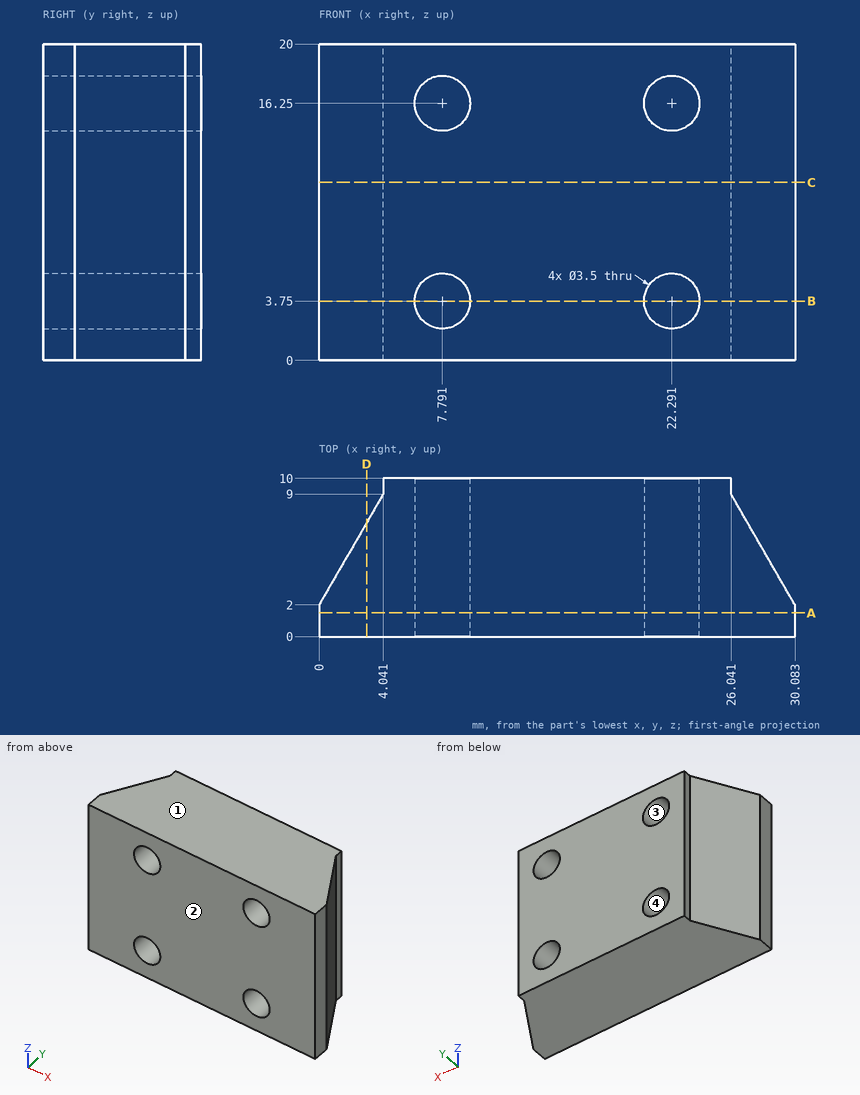
Design review of the part shown in the three views and the two pictorial views. Dimensions are in mm from the part's minimum x, y and z. Round coordinates to 2 decimals unless told otherwise and drop trailing zeros. Write each loop counter-clockwise with the first axis right and the second up, starting at its lowest first coordinate (ties: lowest second). Pieces come first, ordered by that corner, then holes.
Item 1: Consider section D-D on x = 3. Give the boundary of the cut face in (y, z), and give its area (3 significant figures).
Item 2: Consider section B-B on z = 3.75. Give the boundary of the cut face in (x, y).
Item 3: Consider section A-A on y = 1.5. Give the boundary of the cut face in (x, z).
Item 4: Consider section C-C on z = 11.25. Give the boundary of the cut face in (x, y).
Item 5: Draft analysis for pull direction Z (two halves, no side actions). For the marked faces 1, 2, 3 and 4, state which applies: released by +Z, released by -Z, zero draft, split by the parting line, or undercut.
Item 6: For pin 1 Ø3 at (x, z) = (7.79, 3.75) entering from -Y; pin 2 Ø1.1 at (y, z) = (9.5, 5.5) entering from -X; pin 3 Ø0.5 at (y, z) = (9.5, 8.5) entering from +X; pin 4 Ø5 at (y, z) = (7.5, 8.5) entering from -X, all flat-tipped, find the tip position at first contact; note any pin that passes through.
Item 7: Wall thickness on L1, parallel to Z at x = 8, y = 1.5; L2, parallel to X at y = 4, z = 15.75 (1 decimal); L3, parallel to X at y = 9, z = 3.5 (1 decimal): over which ranges is each line inside the solid? List them lowest first.
Check values:
1. outline: (0, 0) - (7.2, 0) - (7.2, 20) - (0, 20) - close
1. area: 144 mm2
2. outline: (0, 0) - (6.04, 0) - (6.04, 10) - (4.04, 10) - (4.04, 9) - (0, 2) - close; (9.54, 0) - (20.54, 0) - (20.54, 10) - (9.54, 10) - close; (24.04, 0) - (30.08, 0) - (30.08, 2) - (26.04, 9) - (26.04, 10) - (24.04, 10) - close
3. outline: (0, 0) - (30.08, 0) - (30.08, 20) - (0, 20) - close; hole circle Ø3.5 at (7.79, 3.75); hole circle Ø3.5 at (7.79, 16.25); hole circle Ø3.5 at (22.29, 3.75); hole circle Ø3.5 at (22.29, 16.25)
4. outline: (0, 0) - (30.08, 0) - (30.08, 2) - (26.04, 9) - (26.04, 10) - (4.04, 10) - (4.04, 9) - (0, 2) - close
5. face 1: released by +Z
5. face 2: zero draft
5. face 3: undercut
5. face 4: undercut
6. pin 1: passes through
6. pin 2: stops at x = 4.01
6. pin 3: stops at x = 26.04
6. pin 4: stops at x = 1.73
7. L1: z = 0 to 2.01, 5.49 to 14.51, 17.99 to 20
7. L2: x = 1.2 to 6.1, 9.5 to 20.6, 24 to 28.9
7. L3: x = 4 to 6.1, 9.5 to 20.6, 24 to 26
